Part model, mm, in its own coordinate system. A direction names the side the tool comes from. Give positions to 0.01 mm unless a question says otherwise; leave off trailing zeros. Write each loop counter-clockwise with the first axis right and the second up, starting at its lowest first coordinate (ties: lowest second). Pieces come first, ordered by that corner, then holes. Notation, with made-up numbers: (15, -30) - (25, -30) arc R34 ccw to (25, 1) - close; hole circle Ø9 at (-1, 35.5). An arc over 180 degrees is marked (long way). Answer as a JSON object with one key per item and string values. Group by question number.
```python
from build123d import *

# Parameters (mm, degrees)
F0_R      = 52.07
F1_DEPTH  = 50.8
F2_R      = 19.05
F5_W      = 25.4
F5_H      = 12.7
F7_DEPTH  = 17.78
F6_W      = 25.4
F6_H      = 12.7
F8_DEPTH  = 17.78
F4_W      = 25.4
F4_H      = 12.7
F9_DEPTH  = 17.78
F3_W      = 25.4
F3_H      = 12.7
F10_DEPTH = 17.78
F0_R_2    = 48.895
F11_DEPTH = 45.72


with BuildPart() as f1:
    # F0 (on Top) → F1 (new body)
    with BuildSketch(Plane.XY):
        with BuildLine():
            Line((59.8627909759, 8.89), (85.2627909759, 8.89))
            ThreePointArc((85.2627909759, 8.89), (60.6167288172, 60.6167288172), (8.89, 85.2627909759))
            Line((8.89, 85.2627909759), (8.89, 59.8627909759))
            Line((8.89, 59.8627909759), (-8.89, 59.8627909759))
            Line((-8.89, 59.8627909759), (-8.89, 85.2627909759))
            ThreePointArc((-8.89, 85.2627909759), (-60.6167288172, 60.6167288172), (-85.2627909759, 8.89))
            Line((-85.2627909759, 8.89), (-59.8627909759, 8.89))
            Line((-59.8627909759, 8.89), (-59.8627909759, -8.89))
            Line((-59.8627909759, -8.89), (-85.2627909759, -8.89))
            ThreePointArc((-85.2627909759, -8.89), (-60.6167288172, -60.6167288172), (-8.89, -85.2627909759))
            Line((-8.89, -85.2627909759), (-8.89, -59.8627909759))
            Line((-8.89, -59.8627909759), (8.89, -59.8627909759))
            Line((8.89, -59.8627909759), (8.89, -85.2627909759))
            ThreePointArc((8.89, -85.2627909759), (60.6167288172, -60.6167288172), (85.2627909759, -8.89))
            Line((85.2627909759, -8.89), (59.8627909759, -8.89))
            Line((59.8627909759, -8.89), (59.8627909759, 8.89))
        make_face()
        Circle(F0_R, mode=Mode.SUBTRACT)
    extrude(amount=F1_DEPTH)

    # F2
    f2_edges = [f1.edges().sort_by_distance(p)[0] for p in [
        (-60.616729, -60.616729, 50.8),
        (60.616729, -60.616729, 50.8),
        (60.616729, 60.616729, 50.8),
        (-60.616729, 60.616729, 50.8),
        (60.616729, -60.616729, 0),
        (60.616729, 60.616729, 0),
        (-60.616729, -60.616729, 0),
        (-60.616729, 60.616729, 0),
    ]]
    fillet(f2_edges, radius=F2_R)

    # F5 (on face) → F7 (join)
    with BuildSketch(Plane(origin=(0, -8.89, 0), x_dir=(-1, 0, 0), z_dir=(0, 1, 0))):
        with Locations((-72.5627909759, 25.4)):
            Rectangle(F5_W, F5_H)
    extrude(amount=F7_DEPTH)

    # F6 (on face) → F8 (join)
    with BuildSketch(Plane(origin=(8.89, 0, 0), x_dir=(0, -1, 0), z_dir=(-1, 0, 0))):
        with Locations((-72.5627909759, 25.4)):
            Rectangle(F6_W, F6_H)
    extrude(amount=F8_DEPTH)

    # F4 (on face) → F9 (join)
    with BuildSketch(Plane.XZ.offset(-8.89)):
        with Locations((-72.5627909759, 25.4)):
            Rectangle(F4_W, F4_H)
    extrude(amount=F9_DEPTH)

    # F3 (on face) → F10 (join)
    with BuildSketch(Plane.YZ.offset(-8.89)):
        with Locations((-72.5627909759, 25.4)):
            Rectangle(F3_W, F3_H)
    extrude(amount=F10_DEPTH)

    # F0 (on Top) → F11 (join)
    with BuildSketch(Plane.XY):
        Circle(F0_R)
        Circle(F0_R_2, mode=Mode.SUBTRACT)
    extrude(amount=F11_DEPTH)


solid = f1.part
```
1) Drop flat-ended pins along their axis: P1, Ø15, axis at y = 73, z = 12, coming from the -X side; P2, Ø19.5, axis at y = 2.5, z = 38.5, coming from the +X side; P3, Ø9, axis at x = 77, y = 1, coming from the -Z side; P4, Ø21, axis at y = -75, z = 40.5, coming from the +X side. Give the stop position or say it passes through.
2) Two-plate mould, pull along X, no slides. Class faces 5 (the flat face through (0, -59.863, 41)), 6 (the flat face through (19, -49, 50.8)), 7 (the flat face through (-8.89, -70, 41)), 8 (the flat face through (85.263, 0, 25)): +X half, -X half, draft (parallel to the pull), parting line (faces both ways), or undercut.
3) Drill centre lines: line 1 along Y through (x, z) = (0, 49.45); line 2 along Y through (x, z) = (1.5, 47.5); line 3 along Z through (x, y) = (-9.5, -51). Where is each one in solid material? Low to high. Write a range as from..to.
4) Saw through at C-C (z = 29). List the corners of the cut face in (x, y) (3 decimals), and give its area (3 significant figures).
5) Saw through at A-A (x = 0). List the corners of the cut face in (y, z) (3 decimals).
6) Saw through at D-D (z = 38.5). List the corners of the cut face in (x, y) (3 decimals).
7) Which spindle directions (+Z, -Z, +X, -X, +Y, -Y) get a long thin tool onto all of the face, cutting with end or side? Do faces 1 (the flat face through (0, -73, 31.75)), 2 (the cylindrical face through (-6.778, 51.627, 48.224)), 3 (the flat face through (59.863, 0, 9)), 4 (the flat face through (-59.863, 0, 9)). Say none if no direction does.
Checks:
{
 "1": {"P1": "x = -53.93", "P2": "x = 85.26", "P3": "z = 19.05", "P4": "x = 54.63"},
 "2": {"face 5": "undercut", "face 6": "draft", "face 7": "undercut", "face 8": "+X half"},
 "3": {"line 1": "-59.86..-52.07, 52.07..59.86", "line 2": "-59.86..-52.05, 52.05..59.86", "line 3": "0..45.72"},
 "4": {"outline": "(-85.263, -8.89) arc R85.725 ccw to (-8.89, -85.263) - (8.89, -85.263) arc R85.725 ccw to (85.263, -8.89) - (85.263, 8.89) arc R85.725 ccw to (8.89, 85.263) - (-8.89, 85.263) arc R85.725 ccw to (-85.263, 8.89) - close; hole circle Ø97.79 at (0, 0)", "area": "15,600 mm2"},
 "5": {"outline": "(-85.263, 19.05) - (-59.863, 19.05) - (-59.863, 0) - (-48.895, 0) - (-48.895, 45.72) - (-52.07, 45.72) - (-52.07, 50.8) - (-59.863, 50.8) - (-59.863, 31.75) - (-85.263, 31.75) - close; (48.895, 0) - (59.863, 0) - (59.863, 19.05) - (85.263, 19.05) - (85.263, 31.75) - (59.863, 31.75) - (59.863, 50.8) - (52.07, 50.8) - (52.07, 45.72) - (48.895, 45.72) - close"},
 "6": {"outline": "(-84.02, -8.89) arc R84.489 ccw to (-8.89, -84.02) - (-8.89, -59.863) - (8.89, -59.863) - (8.89, -84.02) arc R84.489 ccw to (84.02, -8.89) - (59.863, -8.89) - (59.863, 8.89) - (84.02, 8.89) arc R84.489 ccw to (8.89, 84.02) - (8.89, 59.863) - (-8.89, 59.863) - (-8.89, 84.02) arc R84.489 ccw to (-84.02, 8.89) - (-59.863, 8.89) - (-59.863, -8.89) - close; hole circle Ø97.79 at (0, 0)"},
 "7": {"face 1": "+Z, -Y", "face 2": "+Z", "face 3": "-Z, +X", "face 4": "-Z, -X"}
}
